Build history of the part. All positions in model axes, mm. Round coordinates to 2 decimals unless told otherwise and drop trailing zeros. Write each loop counter-clockwise with the first axis right and the second up, starting at its lowest first coordinate (ties: lowest second). Pieces come first, ordered by that corner, then holes. Notation, with made-up numbers: M 26,-4 L 77,-4 A11 cw 77,6 Z; hole C 36,-20 d5. An arc over 180 degrees is marked long. Use a Markdown table: item, result.
from build123d import *

# Parameters (mm, degrees)
F0_W     = 1020
F0_H     = 105
F1_DEPTH = 2
F3_DEPTH = 2
F6_W     = 69.2964494228
F6_H     = 80
F7_DEPTH = 2.001
F8_R     = 5.44999
F9_R     = 2


# Not quite as in the source:
# - a fillet or chamfer is up to 0.001 mm smaller than in the source, because OpenCascade refuses the exact size


with BuildPart() as f1:
    # F0 (on Top) → F1 (new body)
    with BuildSketch(Plane.XY):
        Rectangle(F0_W, F0_H)
    extrude(amount=F1_DEPTH)

    # F2 (on face) → F3 (join)
    with BuildSketch(Plane.XY.offset(2)):
        Polygon((-485, -52.5), (-510, -52.5), (-510, -142.5), (-503, -142.5), (-503, -64.5), (-492.1, -64.5), (-492.1, -142.5), (-485, -142.5), align=None)
    extrude(amount=-F3_DEPTH)

    # F5: F1 across plane


with BuildPart() as f1_1:
    add(f1.part)
    add(f1.part.mirror(Plane.XZ))

    # F6 (on face) → F7 (cut, through all)
    with BuildSketch(Plane.XY.offset(2)):
        with Locations((-500.6258040667, 122.5)):
            Rectangle(F6_W, F6_H)
    extrude(amount=-F7_DEPTH, mode=Mode.SUBTRACT)

    # F8 (radius 5.45 in the source; OpenCascade refuses exactly that, so slightly less here)
    f8_edges = [f1_1.edges().sort_by_distance(p)[0] for p in [
        (-503, -64.5, 1),
        (-492.1, -64.5, 1),
        (-503, 64.5, 1),
        (-492.1, 64.5, 1),
    ]]
    fillet(f8_edges, radius=F8_R)

    # F9
    f9_edges = [f1_1.edges().sort_by_distance(p)[0] for p in [
        (-485, 52.5, 1),
        (-485, 82.5, 1),
        (-492.1, 82.5, 1),
        (-503, 82.5, 1),
        (-510, 82.5, 1),
        (-485, -52.5, 1),
        (-485, -142.5, 1),
        (-492.1, -142.5, 1),
        (-503, -142.5, 1),
        (-510, -142.5, 1),
        (510, -52.5, 1),
        (510, 52.5, 1),
    ]]
    fillet(f9_edges, radius=F9_R)


solid = f1_1.part
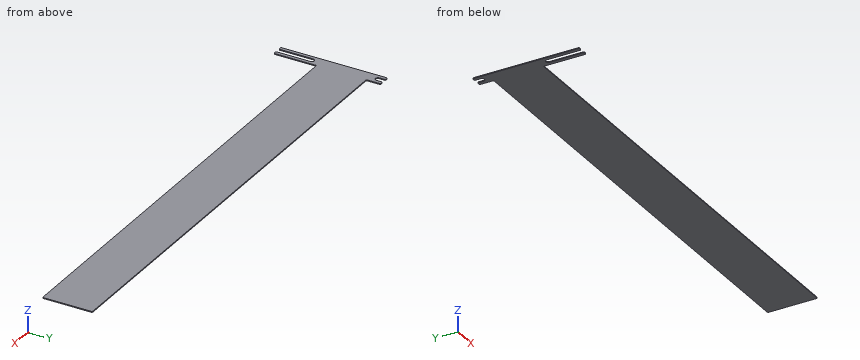
Q1. Cut at A-A on y = -125. Give the cut face in (x, z), and give its area (3 significant figures).
Response values:
| item | result |
|---|---|
| outline | M -510,0 L -503,0 L -503,2 L -510,2 Z; M -492.1,0 L -485,0 L -485,2 L -492.1,2 Z |
| area | 28.2 mm2 |
Q2. Cut at C-C on x = 374. Give the cut face in (y, z).
Response values:
| item | result |
|---|---|
| outline | M -52.5,0 L 52.5,0 L 52.5,2 L -52.5,2 Z |
Q3. Drop a flat-ended pin along its axis: P1, Ø1, axis at y = 74.5, z = 1, coming from the +X side. Give the stop position or say it passes through.
Response values:
| item | result |
|---|---|
| P1 | stops at x = -485 |
Q4. Drill centre lines: L1, parallel to X at y = 72.5, z = 0.65; L2, parallel to X at y = 69, z = 1.4; L3, parallel to Y at x = 107, z = 0.7. Where is each one in solid material? Low to high.
Response values:
| item | result |
|---|---|
| L1 | x = -510 to -503, -492.1 to -485 |
| L2 | x = -510 to -502.92, -492.18 to -485 |
| L3 | y = -52.5 to 52.5 |
